Build history of the part. All positions in model axes, mm. A direction names the side the tool comes from. Give positions to 0.01 mm unless a question says otherwise; leave off trailing zeros. Answer as a JSON object with one key per item and string values. Group by question number.
Q1. Tool access for faces 1 (the flat face through (0, 0, 2)), 2 (the flat face through (-0.13, 13.442, 8.126)), 3 (the flat face through (0.12, 12.77, 18.26)): list every direction of +Z, -Z, +X, -X, +Y, -Y with a clear straight run to the whole face (end or side of a thin tool).
Q2. Drop flat-ended pins along their axis: pin 1 (4 mm diameter, centred on x = 0, z = 10, fed in from -Y); pin 2 (8 mm diameter, centred on x = 7, z = 13, fed in from -Y); pin 3 (5 mm diameter, centred on x = 6, z = 9, fed in from -Y). Give the stop position or say it passes through.
Q3. Two-plate mould, pull along Z, no slides. Class faces 4 (the flat face through (0, 0, 0)), 5 (the flat face through (-2, -12, 30)), 6 (the flat face through (-0.13, -13.351, 9.912)), 7 (the flat face through (-0.25, -12.357, 9.582)): pulls with the +Z half, pulls with the -Z half, needs draft (parallel to the pull), parting line crosses it, or undercut.
Q4. Wall check: probe 1 along Z at (x, y) = (3, 0); probe 2 along X at (y, z) = (3, 14); probe 3 along Y at (x, z) = (4.5, 3.5). Give the ranges that are in metal, low to high. Write a range as from..to.
Q5. Band-saw the part on A-A, the plane x = -6.5. Count the separate pieces of the cut face and the enclosed holes in it, plus the area to 3 significant figures.
from build123d import *

# Parameters (mm, degrees)
SHELL_1_T           = -2
CUT_EXTRUDE_1_DEPTH = 47.230712485
CUT_EXTRUDE_4_DEPTH = 10


with BuildPart() as part:
    # 草图2 → 放样1 section 0
    with BuildSketch(Plane.XY.offset(30)):
        with BuildLine():
            Line((18, -13), (18, 13))
            Line((18, 13), (-18, 13))
            Line((-18, 13), (-18, -13))
            Line((-18, -13), (18, -13))
        make_face()
    # 草图1 → 放样1 section 1
    with BuildSketch(Plane.XY):
        with BuildLine():
            Line((-20, 15), (20, 15))
            Line((20, 15), (20, -15))
            Line((20, -15), (-20, -15))
            Line((-20, -15), (-20, 15))
        make_face()
    loft()

    # 抽壳1
    shell_1_openings = [part.faces().sort_by_distance(p)[0] for p in [
        (0, 0, 30),
    ]]
    offset(amount=SHELL_1_T, openings=shell_1_openings, kind=Kind.INTERSECTION)

    # 草图3 → 切除-拉伸1 (cut, through all)
    with BuildSketch(Plane(origin=(0, -14.933628319, 0.995575221), x_dir=(1, 0, 0), z_dir=(0, -0.997785157856609, 0.06651901052377396))):
        Polygon((9.31271042, 9.002214842), (8.643090631, 19.068807599), (-8.643090631, 19.068807599), (-9.31271042, 9.002214842), align=None)
    extrude(amount=-CUT_EXTRUDE_1_DEPTH, mode=Mode.SUBTRACT)

    # 草图4 → 切除-拉伸4 (cut)
    with BuildSketch(Plane(origin=(19.911504425, 0, 1.327433628), x_dir=(0.066519010523774, 0, -0.997785157856609), z_dir=(0.997785157856609, 0, 0.066519010523774))):
        Polygon((-31.240874648, -6.83151887), (-18.66961979, -7.667746304), (-18.66961979, 8.556289454), (-31.240874648, 7.720062019), align=None)
    extrude(amount=-CUT_EXTRUDE_4_DEPTH, mode=Mode.SUBTRACT)


solid = part.part
Worked answers:
{
 "1": {"face 1": "none", "face 2": "+Y", "face 3": "-Y"},
 "2": {"pin 1": "y = -14.47", "pin 2": "y = -14.4", "pin 3": "y = -14.57"},
 "3": {"face 4": "pulls with the -Z half", "face 5": "pulls with the +Z half", "face 6": "undercut", "face 7": "undercut"},
 "4": {"probe 1": "0..2", "probe 2": "-19.07..-17.06, 17.06..19.07", "probe 3": "-14.77..-12.76, 12.76..14.77"},
 "5": {"separate pieces": "3", "enclosed holes": "0", "area": "132 mm2"}
}
